Work out the finished part from the listing and answer in its coordinate system (mm). Face numbers are marked on the shaded views. A direction names the side the tool comes from. Give positions to 0.01 mm unless a question says otherwise; leave off trailing zeros. Order: outer loops, then holes, each group sorted by start corner. A loop starts at its lowest first (then second) coordinate and runs counter-clockwise, first axis right, second up. Notation, with made-up numbers: (85, -15) - (133, -15) arc R15 cw to (133, 6) - close; hole circle Ø10 at (35, 73.25). An arc over 180 degrees is marked (long way). Write each question's results on one line, items separated by ' | '.
from build123d import *

# Parameters (mm, degrees)
SKETCH1_W                 = 500
SKETCH1_H                 = 113
BOSS_EXTRUDE1_DEPTH       = 5
SKETCH2_W                 = 50
SKETCH2_H                 = 50
BOSS_EXTRUDE3_DEPTH       = 2
LPATTERN1_COUNT           = 2
LPATTERN1_PITCH           = 52
SKETCH3_W                 = 52
SKETCH3_H                 = 51.9
BOSS_EXTRUDE8_DEPTH       = 25
LPATTERN5_COUNT           = 2
LPATTERN5_PITCH           = 52
LPATTERN6_COUNT           = 4
LPATTERN6_PITCH           = 52.1
LPATTERN6_COPY_1_SKETCH_W = 50
LPATTERN6_COPY_1_SKETCH_H = 50
LPATTERN6_COPY_1_DEPTH    = 2
LPATTERN6_COPY_2_SKETCH_W = 50
LPATTERN6_COPY_2_SKETCH_H = 50
LPATTERN6_COPY_2_DEPTH    = 2
LPATTERN6_COPY_3_SKETCH_W = 50
LPATTERN6_COPY_3_SKETCH_H = 50
LPATTERN6_COPY_3_DEPTH    = 2
LPATTERN6_COPY_4_SKETCH_W = 52
LPATTERN6_COPY_4_SKETCH_H = 51.9
LPATTERN6_COPY_4_DEPTH    = 25
LPATTERN6_COPY_5_SKETCH_W = 52
LPATTERN6_COPY_5_SKETCH_H = 51.9
LPATTERN6_COPY_5_DEPTH    = 25
LPATTERN6_COPY_6_SKETCH_W = 52
LPATTERN6_COPY_6_SKETCH_H = 51.9
LPATTERN6_COPY_6_DEPTH    = 25
SKETCH4_W                 = 223.089941366
SKETCH4_H                 = 113
SKETCH4_W_2               = 66.355147464
CUT_EXTRUDE1_DEPTH        = 10


with BuildPart() as part:
    # Sketch1 → Boss-Extrude1 (new body)
    with BuildSketch(Plane(origin=(0, 0, 0), x_dir=(1, 0, 0), z_dir=(0, 1, 0))):
        Rectangle(SKETCH1_W, SKETCH1_H)
    extrude(amount=BOSS_EXTRUDE1_DEPTH)

    # Sketch2 → Boss-Extrude3 (add)
    with BuildSketch(Plane(origin=(0, 5, 0), x_dir=(1, 0, 0), z_dir=(0, 1, 0))):
        with Locations((0, -26.5)):
            Rectangle(SKETCH2_W, SKETCH2_H)
    boss_extrude3 = extrude(amount=BOSS_EXTRUDE3_DEPTH)

    # LPattern1: Boss-Extrude3 ×2
    with Locations(*[(0, 0, -i * LPATTERN1_PITCH) for i in range(1, LPATTERN1_COUNT)]):
        add(boss_extrude3)

    # Sketch3 → Boss-Extrude8 (add)
    with BuildSketch(Plane(origin=(0, 7, 0), x_dir=(1, 0, 0), z_dir=(0, 1, 0))):
        with Locations((0, -26.55)):
            Rectangle(SKETCH3_W, SKETCH3_H)
    boss_extrude8 = extrude(amount=BOSS_EXTRUDE8_DEPTH)

    # LPattern5: Boss-Extrude8 ×2
    with Locations(*[(0, 0, -i * LPATTERN5_PITCH) for i in range(1, LPATTERN5_COUNT)]):
        add(boss_extrude8)

    # LPattern6: Boss-Extrude3, Boss-Extrude8 ×4
    with Locations(*[(i * LPATTERN6_PITCH, 0, 0) for i in range(1, LPATTERN6_COUNT)]):
        add(boss_extrude3)
        add(boss_extrude8)

    # LPattern6 copy 1 sketch → LPattern6 copy 1 (add)
    with BuildSketch(Plane(origin=(52.1, 5, -52), x_dir=(1, 0, 0), z_dir=(0, 1, 0))):
        with Locations((0, -26.5)):
            Rectangle(LPATTERN6_COPY_1_SKETCH_W, LPATTERN6_COPY_1_SKETCH_H)
    extrude(amount=LPATTERN6_COPY_1_DEPTH)

    # LPattern6 copy 2 sketch → LPattern6 copy 2 (add)
    with BuildSketch(Plane(origin=(104.2, 5, -52), x_dir=(1, 0, 0), z_dir=(0, 1, 0))):
        with Locations((0, -26.5)):
            Rectangle(LPATTERN6_COPY_2_SKETCH_W, LPATTERN6_COPY_2_SKETCH_H)
    extrude(amount=LPATTERN6_COPY_2_DEPTH)

    # LPattern6 copy 3 sketch → LPattern6 copy 3 (add)
    with BuildSketch(Plane(origin=(156.3, 5, -52), x_dir=(1, 0, 0), z_dir=(0, 1, 0))):
        with Locations((0, -26.5)):
            Rectangle(LPATTERN6_COPY_3_SKETCH_W, LPATTERN6_COPY_3_SKETCH_H)
    extrude(amount=LPATTERN6_COPY_3_DEPTH)

    # LPattern6 copy 4 sketch → LPattern6 copy 4 (add)
    with BuildSketch(Plane(origin=(52.1, 7, -52), x_dir=(1, 0, 0), z_dir=(0, 1, 0))):
        with Locations((0, -26.55)):
            Rectangle(LPATTERN6_COPY_4_SKETCH_W, LPATTERN6_COPY_4_SKETCH_H)
    extrude(amount=LPATTERN6_COPY_4_DEPTH)

    # LPattern6 copy 5 sketch → LPattern6 copy 5 (add)
    with BuildSketch(Plane(origin=(104.2, 7, -52), x_dir=(1, 0, 0), z_dir=(0, 1, 0))):
        with Locations((0, -26.55)):
            Rectangle(LPATTERN6_COPY_5_SKETCH_W, LPATTERN6_COPY_5_SKETCH_H)
    extrude(amount=LPATTERN6_COPY_5_DEPTH)

    # LPattern6 copy 6 sketch → LPattern6 copy 6 (add)
    with BuildSketch(Plane(origin=(156.3, 7, -52), x_dir=(1, 0, 0), z_dir=(0, 1, 0))):
        with Locations((0, -26.55)):
            Rectangle(LPATTERN6_COPY_6_SKETCH_W, LPATTERN6_COPY_6_SKETCH_H)
    extrude(amount=LPATTERN6_COPY_6_DEPTH)

    # Sketch4 → Cut-Extrude1 (cut)
    with BuildSketch(Plane(origin=(0, 5, 0), x_dir=(1, 0, 0), z_dir=(0, 1, 0))):
        with Locations((-138.455029317, 0)):
            Rectangle(SKETCH4_W, SKETCH4_H)
        with Locations((216.822426268, 0)):
            Rectangle(SKETCH4_W_2, SKETCH4_H)
    extrude(amount=-CUT_EXTRUDE1_DEPTH, mode=Mode.SUBTRACT)


solid = part.part
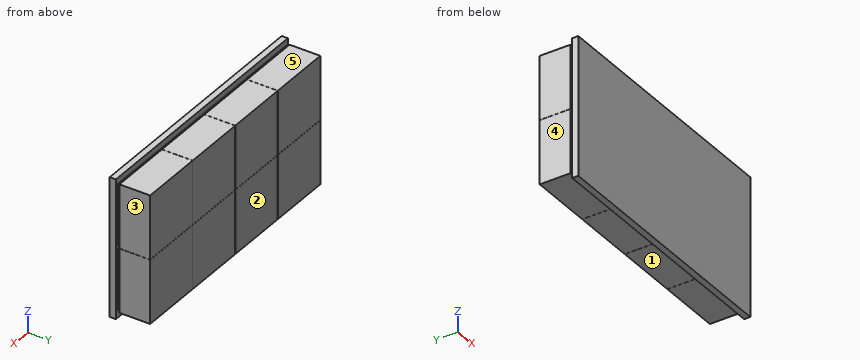
1. A cutting plane is placed at A-A, the plane y = 27. State how many separate pieces and enclosed holes the cut face has, then the cut area to 3 significant figures.
Answer list:
separate pieces: 8 | enclosed holes: 0 | area: 21,600 mm^2
2. Straight lines are drawn through the part: line 1 (Z direction, x = 15, y = 5.5); line 2 (Y direction, x = 131, z = -41). For each, find the intervals that lie inside material, in ascending order. Write a range as [from, to].
Answer list:
line 1: [-50.5, -0.5], [1.5, 51.5] | line 2: [0, 5], [7, 32]
3. A tool of negligible diameter and unlimited length cuts with its end or side. For the marked faces 1, 2, 3, 4 and 5, from which of +Z, -Z, +X, -X, +Y, -Y can it reach the whole face along a straight path? Write none if from no direction.
Answer list:
face 1: -Z, +X, -X, +Y | face 2: +Z, -Z, +X, -X, +Y | face 3: +Z, -Z, +X, +Y | face 4: +Z, -Z, -X, +Y | face 5: +Z, +X, -X, +Y
4. Given P1, Ø7.5, axis at x = 104, y = 21.5, coming from the -Z side; P2, Ø12.5, axis at y = 15.5, z = -21.5, coming from the -X side; P3, Ø1.5, axis at x = 39.5, y = 20.5, coming from the +Z side, each flat-ended and moving along its own axis, determine where each tip first touches the part or whether it passes through.
Answer list:
P1: z = -51.4 | P2: x = -26 | P3: z = 52.5
5. A cutting plane is placed at B-B, the plane x = 8.5. Write down the section's boundary in (y, z), then the cut area to 3 significant figures.
Answer list:
outline: (0, -56.5) - (5, -56.5) - (5, -50.5) - (7, -50.5) - (7, -51.4) - (32, -51.4) - (32, 0.5) - (7, 0.5) - (7, -0.5) - (5, -0.5) - (5, 1.5) - (7, 1.5) - (7, 0.6) - (32, 0.6) - (32, 52.5) - (7, 52.5) - (7, 51.5) - (5, 51.5) - (5, 56.5) - (0, 56.5) - close | area: 3,360 mm^2
